Design review of the part shown in the three views and the two pictorial views. Dimensions are in mm from the part's minimum x, y and z. A direction names the side the tool comes from. Coordinates: 2 decimals unless noted, no trailing zeros. Loops run counter-clockwise (first coordinate to the right, second up) from the corner with the lowest first, then second, coordinate; pieces in that order, holes last.
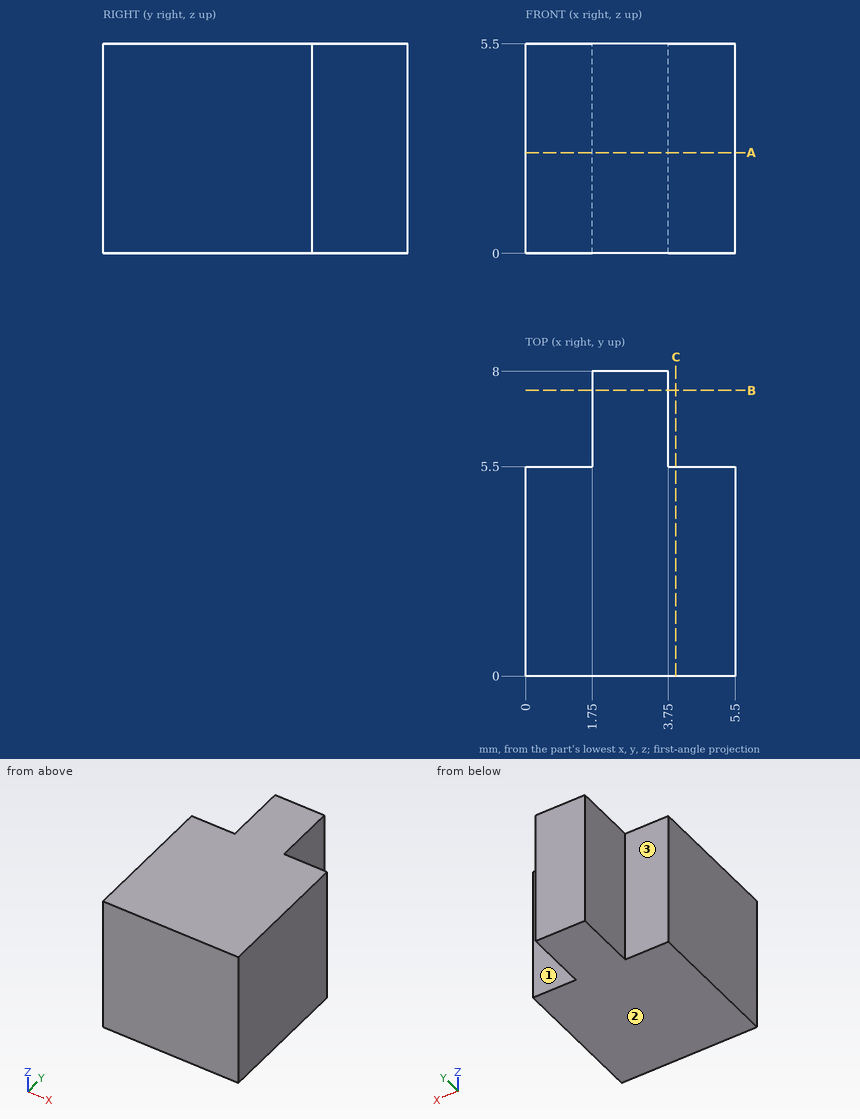
Q1. For pin 1 Ø1.9 at (x, z) = (0.5, 2.5) entering from +Y, flat-tipped, find the tip position at first contact; note if it passes through.
Q2. Consider section A-A (z = 2.65). State the section outline as (x, y) points, then the cut area to 4 significant figures.
Q3. Consider section C-C (x = 3.95). State the section outline as (y, z) points, then the cut area to 4 significant figures.
Q4. Wall thickness on probe 1 along X at (y, z) = (7.75, 1.2); probe 2 along Y at (x, z) = (1.2, 2.9): over which ranges is each line inside the solid? List them lowest first.
Q5. Machinability: for the marked faces 1, 2 and 3, which of the approach directions +Z, -Z, +X, -X, +Y, -Y give a long, thin tool a straight path to every point of the face, cutting with its end or side? Answer none if there is none.
Q6. Consider section B-B (y = 7.5). State the section outline as (x, z) points.
Model answer:
1. pin 1: stops at y = 5.5
2. outline: (0, 0) - (5.5, 0) - (5.5, 5.5) - (3.75, 5.5) - (3.75, 8) - (1.75, 8) - (1.75, 5.5) - (0, 5.5) - close
2. area: 35.25 mm2
3. outline: (0, 0) - (5.5, 0) - (5.5, 5.5) - (0, 5.5) - close
3. area: 30.25 mm2
4. probe 1: x = 1.75 to 3.75
4. probe 2: y = 0 to 5.5
5. face 1: +Z, -Z, +X, +Y
5. face 2: -Z, +X, -X, +Y, -Y
5. face 3: +Z, -Z, -X, +Y
6. outline: (1.75, 0) - (3.75, 0) - (3.75, 5.5) - (1.75, 5.5) - close
